Solid Edge part; units mm, degrees
sketch "Sketch1" plane through (0, 0, 0) normal (0, -1, 0) x (1, 0, 0)
  line L0 (-45, -40) -> (45, -40)
  line L1 (45, -40) -> (45, 40)
  line L2 (45, 40) -> (-45, 40)
  line L3 (-45, 40) -> (-45, -40)
  dimension "D1" = 45
  dimension "D2" = 45
extrude "Protrusion1" add sketch "Sketch1" along normal mid plane 5
sketch "Sketch2" plane through (35, -2.5, 0) normal (0, -1, 0) x (-1, 0, 0)
  circle A0 centre (-5, 30) radius 2.25
  circle A1 centre (75, 30) radius 2.25
  circle A2 centre (75, -30) radius 2.25
  circle A3 centre (-5, -30) radius 2.25
extrude "Cutout1" cut sketch "Sketch2" against normal through all
sketch "Sketch3" plane through (0, -2.5, 0) normal (0, -1, 0) x (-1, 0, 0)
  line L0 (-30, 40) -> (-25, 40)
  line L1 (-25, 40) -> (-25, -40)
  line L2 (-25, -40) -> (-30, -40)
  line L3 (-30, -40) -> (-30, 40)
  dimension "D1" = 30
extrude "Extrusionsausprägung_26" add sketch "Sketch3" along normal blind 40
sketch "Sketch4" plane through (0, -20, -40) normal (0, 0, -1) x (-1, 0, 0)
  line L0 (-25, 17.5) -> (-20, 17.5)
  line L1 (-20, 17.5) -> (-20, 12.5)
  line L2 (-20, 12.5) -> (-24.3301, 5)
  line L3 (-24.3301, 5) -> (-20, -2.5)
  line L4 (-20, -2.5) -> (-20, -22.5)
  line L5 (-20, -22.5) -> (-25, -22.5)
  line L6 (-25, -22.5) -> (-25, 17.5)
  dimension "D1" = 25
  dimension "D2" = 20
extrude "Protrusion2" add sketch "Sketch4" against normal up to vertex (80 mm away)
sketch "Sketch5" plane through (-12.5, -2.5, 0) normal (0, -1, 0) x (-1, 0, 0)
  circle A0 centre (21, 0) radius 1.875
  dimension "D1" = 21
extrude "Cutout2" cut sketch "Sketch5" against normal through all
sketch "Sketch6" plane through (20, -32.5, 0) normal (-1, 0, 0) x (0, 1, 0)
  circle A0 centre (-4.95, 30) radius 1.875
  circle A1 centre (-4.95, -30) radius 1.875
  dimension "D1" = 4.95
extrude "Cutout3" cut sketch "Sketch6" against normal through all
sketch "Sketch7" plane through (30, -22.5, 0) normal (1, 0, 0) x (0, -1, 0)
  line L0 (20, 5) -> (-10, 5)
  line L1 (-10, 5) -> (-10, 0)
  line L2 (-10, 0) -> (20, 0)
  line L3 (20, 0) -> (20, 5)
  dimension "D1" = 20
  dimension "D2" = 20
extrude "Extrusionsausprägung_28" add sketch "Sketch7" along normal blind 25
sketch "Sketch8" plane through (42.5, -27.5, -5) normal (0, 0, -1) x (-1, 0, 0)
  circle A0 centre (-3.299, 9) radius 1.4
  circle A1 centre (-3.299, -9) radius 1.4
  dimension "D1" = 3.299
extrude "Cutout4" cut sketch "Sketch8" against normal through all
chamfer "Fase_6" distance 0.5 angle 45 7 edges at (42.25, -2.5, -30) (42.25, -2.5, 30) (-37.75, -2.5, -30) (-37.75, -2.5, 30) (-31.625, -2.5, 0) (20, -39.325, 30) (20, -39.325, -30)
chamfer "Fase_7" distance 0.3 angle 45 2 edges at (47.199, -18.5, 0) (47.199, -36.5, 0)
fillet "Verrundung_6" radius 5 6 edges at (45, -2.5, 0) (-45, -2.5, 0) (30, -27.5, -5) (30, -27.5, 0) (30, -22.5, -40) (30, -22.5, 40)
properties part number "A7.2" material "Nylon, allgemein"
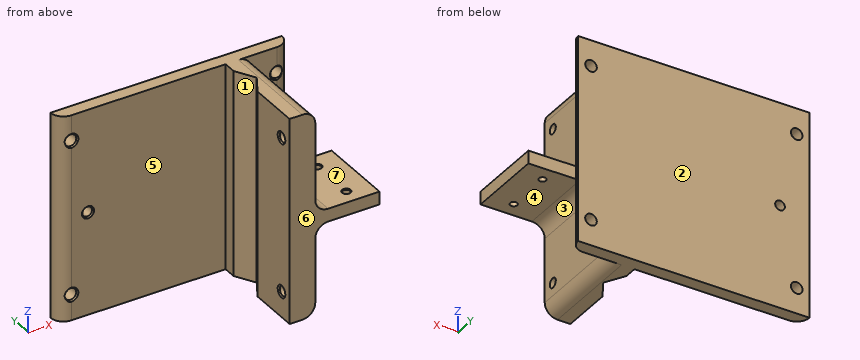
Could you check a few things on this model? Use its own coordinates, in mm. Face numbers are marked on the shaded views. A direction names the side the tool comes from. Give positions to 0.01 mm unless a question says otherwise; leave off trailing zeros. Order: outer loops, then holes, each group sorted by start corner. A loop starts at its lowest first (then second) coordinate and runs counter-clockwise, first axis right, second up.
Q1. Suppose I cut it at B-B, the plane z = -20. Write out the boundary of the cut face in (x, y), and give its area (3 significant figures).
Q2. Suppose I cut it at D-D, the plane x = -5.5. Write out the boundary of the cut face in (y, z), and give its area (3 significant figures).
Q3. We'd pull the mould along Y, two halves only. Please class the marked faces 1, 2 and 3: +Y half, -Y half, draft (parallel to the pull), parting line (faces both ways), or undercut.
Q4. If I drill on line 1 along Z through (x, y) = (-40, 1.4); line 2 along Y through (x, z) = (28.25, 30) (3 decimals); line 3 along X through (y, z) = (-0.7, -30), over which ranges is the centre line in solid material (lowest first)?
Q5. For the marked faces 4, 5, 6 and 7, which set-ups out of +Z, -Z, +X, -X, +Y, -Y let a thin tool reach every point of the face, with its end or its side?
Q6. Suppose I cut it at A-A, the plane y = -33.5. Write out the boundary of the cut face in (x, z), and give its area (3 significant figures).
Q7. Suppose I cut it at C-C, the plane y = -18.5. Write out the boundary of the cut face in (x, z), and give its area (3 significant figures).
Q8. I'm going to push flat-ended pins straight in: P1, Ø3, axis at x = 45.799, y = -36.5, coming from the -Z side; P2, Ø2.5, axis at x = -40, z = 30, coming from the +Y side; P3, Ø12, axis at y = -17.5, z = 27, coming from the -X side; P4, Ø4, axis at x = 29, y = -11, coming from the +Z side. Where does each tip first touch, or does it pass through?
Solution:
1. outline: (-45, 2.5) arc R5 ccw to (-40, -2.5) - (20, -2.5) - (20, -7.5) - (24.33, -15) - (20, -22.5) - (20, -42.5) - (30, -42.5) - (30, -2.5) - (40, -2.5) arc R5 ccw to (45, 2.5) - close
1. area: 807 mm2
2. outline: (-2.5, -40) - (2.5, -40) - (2.5, 40) - (-2.5, 40) - close
2. area: 400 mm2
3. face 1: undercut
3. face 2: +Y half
3. face 3: draft
4. line 1: z = -40 to -32.25, -27.75 to 27.75, 32.25 to 40
4. line 2: y = -42.5 to -39.325, -35.575 to 2.5
4. line 3: x = -43.84 to -42.25, -37.75 to 37.75, 42.25 to 43.84
5. face 4: -Z, +X, -Y
5. face 5: +Z, -Z, -X, -Y
5. face 6: +Z, -Z, +X, -X, -Y
5. face 7: +Z, +X, -Y
6. outline: (20, -40) - (25, -40) arc R5 ccw to (30, -35) - (30, -10) arc R5 cw to (35, -5) - (55, -5) - (55, 0) - (35, 0) arc R5 cw to (30, 5) - (30, 35) arc R5 ccw to (25, 40) - (20, 40) - close
6. area: 925 mm2
7. outline: (22.31, -40) - (25, -40) arc R5 ccw to (30, -35) - (30, -10) arc R5 cw to (35, -5) - (44.4, -5) - (44.4, -0.3) - (44.1, 0) - (35, 0) arc R5 cw to (30, 5) - (30, 35) arc R5 ccw to (25, 40) - (22.31, 40) - close; (47.2, -5) - (55, -5) - (55, 0) - (47.5, 0) - (47.2, -0.3) - close
7. area: 726 mm2
8. P1: stops at z = -5
8. P2: passes through
8. P3: stops at x = 20
8. P4: stops at z = 39.58
